Autodesk Inventor part; units mm, degrees
ref_plane "YZ Plane" through (0, 0, 0) normal (1, 0, 0) x (0, 1, 0)
ref_plane "XZ Plane" through (0, 0, 0) normal (0, 1, 0) x (-1, 0, 0)
ref_plane "XY Plane" through (0, 0, 0) normal (0, 0, 1) x (1, 0, 0)
sketch "Sketch1" plane through (0, 0, 0) normal (0, 0, 1) x (1, 0, 0)
  line L0 (-4.7637, 0) -> (8.2363, 0)
  line L1 (8.2363, 0) -> (8.2363, 13)
  line L2 (8.2363, 13) -> (-4.7637, 13)
  line L3 (-4.7637, 13) -> (-4.7637, 0)
  arc A0 (-4.7637, 0) -> (-0.7637, 13) centre (-33.6274, 15.9965) ccw
  arc A1 (4.2363, 13) -> (8.2363, 0) centre (37.1, 15.9965) ccw
  point P0 (0, 0)
  dimension "d0" = 13
  dimension "d1" = 13
  dimension "d2" = 4
  dimension "d3" = 4
  dimension "d4" = 33
  dimension "d5" = 33
extrude "Extrusion1" add sketch "Sketch1" along normal blind 25 contours A0 L2 A1 L0
sketch "Sketch2" plane through (-4.7637, 0, 0) normal (0, -1, 0) x (1, 0, 0)
  line L0 (3.9, 20.185) -> (9.1, 20.185)
  line L1 (9.1, 20.185) -> (9.1, 18.585)
  line L2 (9.1, 18.585) -> (3.9, 18.585)
  line L3 (3.9, 18.585) -> (3.9, 20.185)
  line L4 (3.9, 6.415) -> (9.1, 6.415)
  line L5 (9.1, 6.415) -> (9.1, 4.815)
  line L6 (9.1, 4.815) -> (3.9, 4.815)
  line L7 (3.9, 4.815) -> (3.9, 6.415)
  line L8 (0, 0) -> (0, 25)
  line L9 (0, 25) -> (13, 25)
  point P0 (4.7637, 0)
  dimension "d8" = 5.2
  dimension "d9" = 3.9
  dimension "d10" = 1.6
  dimension "d11" = 1.6
  dimension "d12" = 15.37
  dimension "d13" = 4.815
  dimension "d23" = 13
extrude "Extrusion2" cut sketch "Sketch2" against normal blind 2
fillet "Fillet1" radius 1 8 edges at (4.2363, 13, 12.5) (1.7363, 13, 25) (-0.7637, 13, 12.5) (1.7363, 13, 0) (5.5593, 6.2917, 25) (-2.0867, 6.2917, 25) (5.5593, 6.2917, 0) (-2.0867, 6.2917, 0)
sketch "Sketch4" plane through (-4.7637, 2, 0) normal (0, -1, 0) x (1, 0, 0)
  point P0 (4.7637, 0)
sketch "Sketch5" plane through (-4.7637, 2, 0) normal (0, -1, 0) x (1, 0, 0)
  line L0 (3.9, 18.585) -> (9.1, 18.585)
  line L1 (8.6, 19.985) -> (4.4, 19.985)
  line L2 (4.4, 19.985) -> (4.4, 18.585)
  line L3 (4.4, 18.585) -> (8.6, 18.585)
  line L4 (8.6, 18.585) -> (8.6, 19.985)
  line L5 (3.9, 18.585) -> (3.9, 20.185)
  line L6 (9.1, 20.185) -> (9.1, 18.585)
  line L7 (9.1, 6.415) -> (3.9, 6.415)
  line L8 (4.4, 6.415) -> (8.6, 6.415)
  line L9 (8.6, 6.415) -> (8.6, 4.9558)
  line L10 (8.6, 4.9558) -> (4.4, 4.9558)
  line L11 (4.4, 4.9558) -> (4.4, 6.415)
  point P0 (4.7637, 0)
  dimension "d24" = 1.4
  dimension "d25" = 0.5
  dimension "d26" = 0.5
extrude "Extrusion4" cut sketch "Sketch5" against normal blind 10
properties part number "DoubleSliderCap"
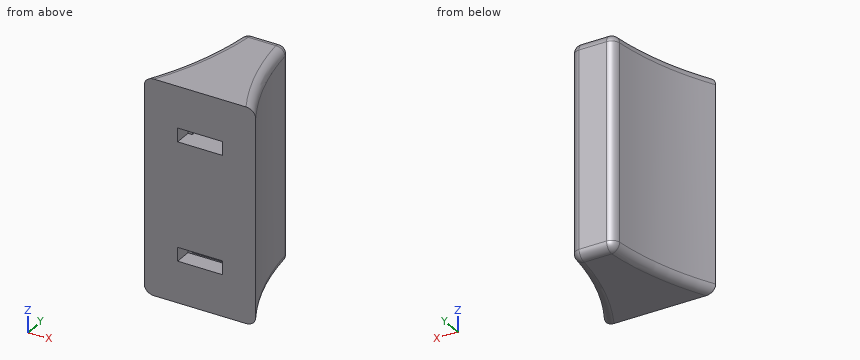
Here's how the part is built. I have some questions about the finished solid (model axes, mm). Coordinates: 2 decimals unless noted, no trailing zeros. Write each loop counter-clockwise with the first axis right and the second up, starting at its lowest first coordinate (ties: lowest second). Pieces come first, ordered by that corner, then holes.
Item 1: Will these pins go through, and if not, where does the flat tip stop? pin 1 (2 mm diameter, centred on y = 11, z = 9, fed in from -X); pin 2 (1 mm diameter, centred on y = 3.5, z = 10, fed in from +X); pin 3 (0.5 mm diameter, centred on y = 1.5, z = 19, fed in from -X).
Item 2: I want a section at A-A on x = 2. Write out the boundary of the cut face in (y, z) (3 decimals).
Item 3: If I drill on line 1 (Z direction, x = 0.5, y = 1.5) (3 decimals); line 2 (Z direction, x = 1.25, y = 2.75) (3 decimals); line 3 (Y direction, x = 1.75, z = 19.5), over which ranges is the centre line in solid material (lowest first)?
Item 4: I want a section at B-B on z = 4.25. Write out the boundary of the cut face in (x, y).
Item 5: I want a section at C-C on y = 2.5. Count the separate pieces of the cut face and the enclosed holes in it, and give its area (3 significant figures).
Findings below:
1. pin 1: stops at x = -1.18
1. pin 2: stops at x = 6.77
1. pin 3: stops at x = -4.11
2. outline: (0, 0) - (12, 0) arc R1 ccw to (13, 1) - (13, 24) arc R1 ccw to (12, 25) - (0, 25) - (0, 20.185) - (2, 20.185) - (2, 19.985) - (12, 19.985) - (12, 18.585) - (0, 18.585) - (0, 6.415) - (12, 6.415) - (12, 4.956) - (2, 4.956) - (2, 4.815) - (0, 4.815) - close
3. line 1: z = 0 to 4.815, 6.415 to 18.585, 20.185 to 25
3. line 2: z = 0 to 4.956, 6.415 to 18.585, 19.985 to 25
3. line 3: y = 12 to 13
4. outline: (-4.76, 0) - (8.24, 0) arc R33 cw to (4.33, 12.12) arc R1 ccw to (3.34, 13) - (0.14, 13) arc R1 ccw to (-0.86, 12.12) arc R33 cw to start
5. separate pieces: 1
5. enclosed holes: 2
5. area: 250 mm2
